Autodesk Inventor part; units mm, degrees
ref_plane "Work Plane1" through (-29.1, -14.5, 2.4) normal (0, 0, -1) x (0, 1, 0)
ref_plane "Work Plane2" through (-13.8999, -10.5497, 2.25) normal (0, 0, -1) x (0, 1, 0)
ref_plane "YZ Plane" through (0, 0, 0) normal (1, 0, 0) x (0, 1, 0)
ref_plane "Work Plane1" through (-29.1, -14.5, 2.4) normal (0, 0, -1) x (0, 1, 0)
ref_plane "Work Plane2" through (-13.8999, -10.5497, 2.25) normal (0, 0, -1) x (0, 1, 0)
sketch "Sketch1" plane through (0, 0, 0) normal (0, 0, 1) x (1, 0, 0)
  line L0 (-34.86, 0) -> (34.86, 0) construction
  line L1 (0, -34.86) -> (0, 34.86) construction
  line L2 (0, 0) -> (11.1575, 11.1575) construction
  line L3 (0, 0) -> (15.7791, 0) construction
  line L4 (0, 24.9) -> (16.8009, 24.9)
  line L5 (16.8009, 24.9) -> (16.8009, 21.2415)
  line L6 (16.8009, 21.2415) -> (19.0212, 19.0212)
  line L7 (24.9, 0) -> (24.9, 16.8009)
  line L8 (24.9, 16.8009) -> (21.2415, 16.8009)
  line L9 (21.2415, 16.8009) -> (19.0212, 19.0212)
  line L10 (0, -24.9) -> (16.8009, -24.9)
  line L11 (16.8009, -24.9) -> (16.8009, -21.2415)
  line L12 (16.8009, -21.2415) -> (19.0212, -19.0212)
  line L13 (24.9, 0) -> (24.9, -16.8009)
  line L14 (24.9, -16.8009) -> (21.2415, -16.8009)
  line L15 (21.2415, -16.8009) -> (19.0212, -19.0212)
  line L16 (0, 24.9) -> (-16.8009, 24.9)
  line L17 (-16.8009, 24.9) -> (-16.8009, 21.2415)
  line L18 (-16.8009, 21.2415) -> (-19.0212, 19.0212)
  line L19 (-24.9, 16.8009) -> (-21.2415, 16.8009)
  line L20 (-21.2415, 16.8009) -> (-19.0212, 19.0212)
  line L21 (0, -24.9) -> (-16.8009, -24.9)
  line L22 (-16.8009, -24.9) -> (-16.8009, -21.2415)
  line L23 (-16.8009, -21.2415) -> (-19.0212, -19.0212)
  line L24 (-21.2415, -16.8009) -> (-19.0212, -19.0212)
  line L25 (-24.9, -16.8009) -> (-21.2415, -16.8009)
  line L26 (-24.9, 0) -> (-24.9, -16.8009)
  line L27 (-24.9, 0) -> (-24.9, 16.8009)
  circle A0 centre (0, 0) radius 10
  dimension "d0" = 45
  dimension "d2" = 24.9
  dimension "d3" = 3.14
  dimension "d4" = 26.9
  dimension "d5" = 20
extrude "Extrusion1" add sketch "Sketch1" along normal up to surface (2.25 mm away)
sketch "Sketch5" plane through (0, 0, 0) normal (0, 0, -1) x (-1, 0, 0)
  circle A0 centre (-9.7, 10) radius 1.4
  circle A1 centre (-9.7, -10) radius 1.4
  circle A2 centre (13.8, 0) radius 1.4
  circle A3 centre (-10, 6.9) radius 0.75
  circle A4 centre (10, 6.9) radius 1.25
  point P0 (0, 0)
hole "Hole1" at (-13.8, 0, 0) at (9.7, -10, 0) at (-10, 6.9, 0) at (9.7, 10, 0) direction (0, 0, 1) diameter 3.3 depth 12 tip angle 118
sketch "Skizze6" plane through (-16.8009, 24.9, 2.25) normal (0, 0, 1) x (1, 0, 0)
  circle A0 centre (6.8009, -18) radius 1.65 construction
  circle A1 centre (3.0009, -24.9) radius 1.65 construction
  circle A2 centre (26.5009, -34.9) radius 1.65 construction
  circle A3 centre (26.5009, -14.9) radius 1.65 construction
  circle A4 centre (16.8009, -24.9) radius 10 construction
  line L0 (33.6017, -3.6585) -> (33.6017, 0)
  line L1 (33.6017, 0) -> (0, 0) construction
  line L2 (0, 0) -> (0, -3.6585)
  line L3 (0, -3.6585) -> (-4.4406, -8.0991)
  line L4 (-4.4406, -8.0991) -> (-8.0991, -8.0991)
  line L5 (-8.0991, -8.0991) -> (-8.0991, -41.7009) construction
  line L6 (-8.0991, -41.7009) -> (-4.4406, -41.7009)
  line L7 (-4.4406, -41.7009) -> (0, -46.1415)
  line L8 (0, -46.1415) -> (0, -49.8)
  line L9 (0, -49.8) -> (33.6017, -49.8) construction
  line L10 (33.6017, -49.8) -> (33.6017, -46.1415)
  line L11 (33.6017, -46.1415) -> (38.0423, -41.7009)
  line L12 (38.0423, -41.7009) -> (41.7009, -41.7009)
  line L13 (41.7009, -41.7009) -> (41.7009, -8.0991) construction
  line L14 (41.7009, -8.0991) -> (38.0423, -8.0991)
  line L15 (38.0423, -8.0991) -> (33.6017, -3.6585)
  line L16 (-0.1, 0.1) -> (33.7017, 0.1) construction
  line L17 (33.7017, 0.1) -> (33.7017, -3.6171)
  line L18 (33.7017, -3.6171) -> (38.0838, -7.9991)
  line L19 (38.0838, -7.9991) -> (41.8009, -7.9991)
  line L20 (41.8009, -7.9991) -> (41.8009, -41.8009) construction
  line L21 (41.8009, -41.8009) -> (38.0838, -41.8009)
  line L22 (38.0838, -41.8009) -> (33.7017, -46.1829)
  line L23 (33.7017, -46.1829) -> (33.7017, -49.9)
  line L24 (33.7017, -49.9) -> (-0.1, -49.9) construction
  line L25 (-0.1, -49.9) -> (-0.1, -46.1829)
  line L26 (-0.1, -46.1829) -> (-4.4821, -41.8009)
  line L27 (-4.4821, -41.8009) -> (-8.1991, -41.8009)
  line L28 (-8.1991, -41.8009) -> (-8.1991, -7.9991) construction
  line L29 (-8.1991, -7.9991) -> (-4.4821, -7.9991)
  line L30 (-4.4821, -7.9991) -> (-0.1, -3.6171)
  line L31 (-0.1, -3.6171) -> (-0.1, 0.1)
  line L32 (-8.0991, -8.0991) -> (-8.0991, -7.9991)
  line L33 (0, 0) -> (-0.1, 0)
  line L34 (33.6017, 0) -> (33.7017, 0)
  line L35 (41.7009, -8.0991) -> (38.0423, -8.0991)
  line L36 (41.7009, -8.0991) -> (41.7009, -7.9991)
  line L37 (41.7009, -41.7009) -> (41.7009, -41.8009)
  line L38 (33.6017, -49.8) -> (33.7017, -49.8)
  line L39 (-8.0991, -41.7009) -> (-8.0991, -41.8009)
  line L40 (0, -49.8) -> (-0.1, -49.8)
  point P0 (16.8009, -24.9)
  dimension "d25" = 0.1
extrude "IM_offset" add sketch "Skizze6" against normal up to surface (2.25 mm away)
properties part number "20_Cube_insert_AlliedVision_Alvium_v3"
The listing builds one solid part. Answer for the finished solid, in the listing's coordinates (mm). A direction names the side the tool comes from. Give positions to 0.01 mm unless a question says otherwise; leave off trailing zeros. Order: outer loops, then holes, each group sorted by start corner. A loop starts at its lowest first (then second) coordinate and runs counter-clockwise, first axis right, second up. Notation, with made-up numbers: (-26, 16.25) -> (2, 16.25) arc R27 cw to (2, 33.25) -> close; hole circle Ø4 at (-31.5, -18.75). An arc over 180 degrees is marked (long way). Write each question's results on one line, items separated by ' | '.
Q1. The part is cut by section A-A, the plane y = 0. Give the vertices of the cut face in (x, z), and give its area (3 significant figures).
Checked values:
outline: (-24.9, 0) -> (-15.45, 0) -> (-15.45, 2.25) -> (-24.9, 2.25) -> close; (-12.15, 0) -> (-10, 0) -> (-10, 2.25) -> (-12.15, 2.25) -> close; (10, 0) -> (24.9, 0) -> (24.9, 2.25) -> (10, 2.25) -> close | area: 59.6 mm^2
Q2. The part is cut by section C-C, the plane z = 1.25. Give the vertices of the cut face in (x, y), and give its area (3 significant figures).
Checked values:
outline: (-24.9, -16.9) -> (-21.28, -16.9) -> (-16.9, -21.28) -> (-16.9, -24.9) -> (16.9, -24.9) -> (16.9, -21.28) -> (21.28, -16.9) -> (24.9, -16.9) -> (24.9, 16.9) -> (21.28, 16.9) -> (16.9, 21.28) -> (16.9, 24.9) -> (-16.9, 24.9) -> (-16.9, 21.28) -> (-21.28, 16.9) -> (-24.9, 16.9) -> close; hole circle Ø3.3 at (-13.8, 0); hole circle Ø3.3 at (-10, 6.9); hole circle Ø20 at (0, 0); hole circle Ø3.3 at (9.7, -10); hole circle Ø3.3 at (9.7, 10) | area: 1,910 mm^2
Q3. Straight lines are drawn through the part: probe 1 along Y at (x, z) = (-9, 0.65); probe 2 along Y at (x, z) = (-13.8, 1.55); probe 3 along X at (y, z) = (5.5, 0.85). For each, find the intervals that lie inside material, in ascending order. Write a range as from..to.
Checked values:
probe 1: y = -24.9..-4.36, 4.36..5.59, 8.21..24.9 | probe 2: y = -24.9..-1.65, 1.65..24.9 | probe 3: x = -24.9..-10.87, -9.13..-8.35, 8.35..24.9
Q4. The part is cut by section D-D, the plane y = -7.5. Give the vertices of the cut face in (x, z).
Checked values:
outline: (-24.9, 0) -> (-6.61, 0) -> (-6.61, 2.25) -> (-24.9, 2.25) -> close; (6.61, 0) -> (24.9, 0) -> (24.9, 2.25) -> (6.61, 2.25) -> close
Q5. Which of the six approach directions +Z, -Z, +X, -X, +Y, -Y give full straight-line access (tool end or side, diameter ignored) to faces 1 (the face through (-16.901, 23, 1)), 2 (the face through (16.901, 23, 1)), 3 (the face through (-23, -16.901, 1)), 4 (the face through (23, -16.901, 1))?
Checked values:
face 1: +Z, -Z, -X, +Y | face 2: +Z, -Z, +X, +Y | face 3: +Z, -Z, -X, -Y | face 4: +Z, -Z, +X, -Y
Q6. The part is cut by section B-B, the plane x = 0. Give the vertices of the cut face in (y, z).
Checked values:
outline: (-24.9, 0) -> (-10, 0) -> (-10, 2.25) -> (-24.9, 2.25) -> close; (10, 0) -> (24.9, 0) -> (24.9, 2.25) -> (10, 2.25) -> close
